Geometry: see drawing. Coordinates: mm, zero at the bounding-box minimum. A direction names the side the tool comes from. Give positions to 0.01 mm unless a question says otherwise; leave off trailing zeros. Write each loop counter-clockwise with the first axis right and the second up, starting at its lowest first coordinate (ties: lowest second). Pieces come first, ordered by that corner, then holes.
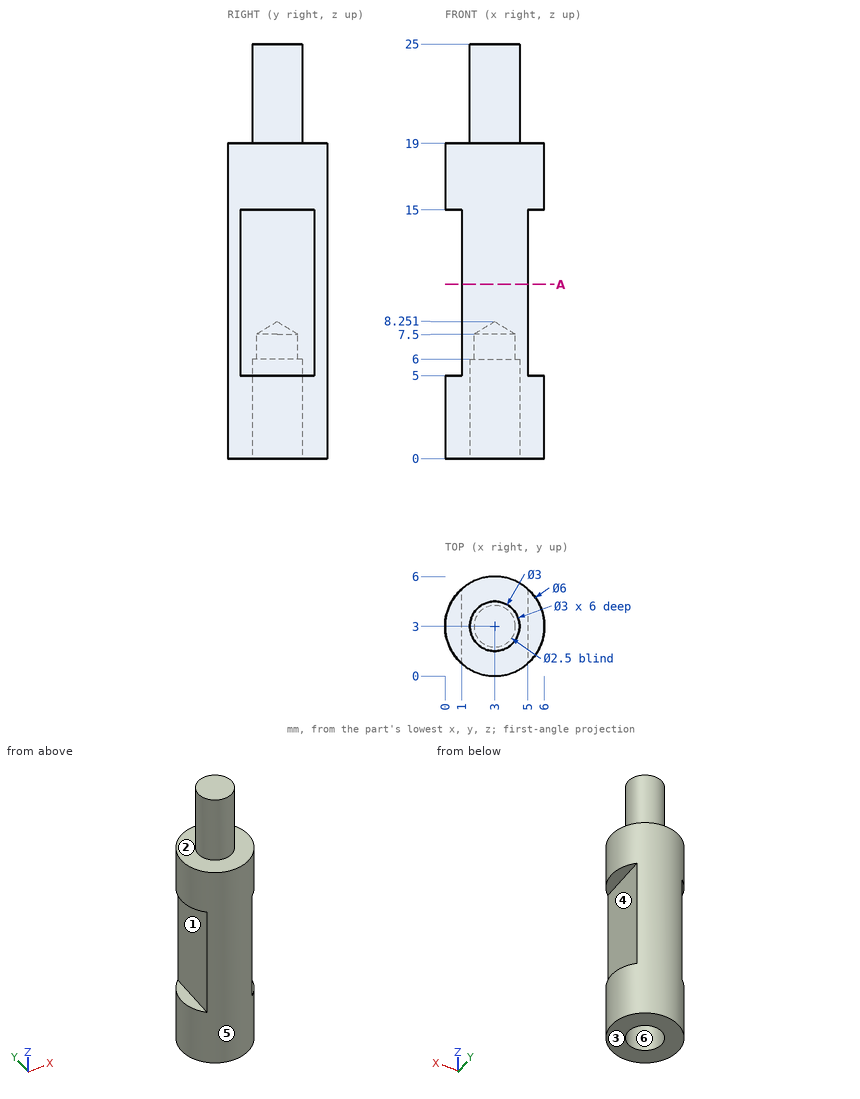
1. Pin query (flat end, axial travel): P1, Ø1.1, axis at x = 0.5, y = 2.5, coming from the -Z side; P2, Ø2, axis at y = 5, z = 3.5, coming from the +X side; P3, Ø0.9, axis at x = 3.5, y = 3, coming from the -Z side; P4, Ø0.8, axis at x = 0.5, y = 2.5, coming from the +Z side. Return the tip coordinate at first contact, or that it passes through.
2. Line query: probe 1 along Z at (x, y) = (5.5, 1.7); probe 2 along Y at (x, z) = (3, 6.5); probe 3 along Y at (x, z) = (3, 1.9). Output: solid intervals per line, ascending.
3. Access query for the marked faces 1, 2 and 3. Directions: +Z, -Z, +X, -X, +Y, -Y. A direction counts if a zero-diameter tool reaches every point of the face in a straight line with its end or side. Return the directions, or none.
4. Pull-direction query (Y, two-part tool) for the marked faces 4, 5 and 6; classes: pulls with the +Y half, pulls with the -Y half, needs draft (parallel to the pull), parting line crosses it, or undercut.
5. Section query A-A (z = 10.5). Return loops of the section in (x, y), plus the area to 3 significant figures.
The answers:
1. P1: stops at z = 0
1. P2: stops at x = 5.83
1. P3: stops at z = 7.68
1. P4: stops at z = 19
2. probe 1: z = 0 to 5, 15 to 19
2. probe 2: y = 0 to 1.75, 4.25 to 6
2. probe 3: y = 0 to 1.5, 4.5 to 6
3. face 1: -X, +Y, -Y
3. face 2: +Z
3. face 3: -Z, +X, -X, +Y, -Y
4. face 4: needs draft
4. face 5: parting line crosses it
4. face 6: undercut
5. outline: (1, 0.76) arc R3 ccw to (5, 0.76) - (5, 5.24) arc R3 ccw to (1, 5.24) - close
5. area: 22.1 mm2
